from build123d import *

# Parameters (mm, degrees)
SKETCH1_R           = 3
BOSS_EXTRUDE1_DEPTH = 2
FILLET1_R           = 2


with BuildPart() as part:
    # Sketch1 → Boss-Extrude1 (new, symmetric)
    with BuildSketch(Plane(origin=(0, 0, 0), x_dir=(1, 0, 0), z_dir=(0, 1, 0))):
        with BuildLine():
            Line((0, -7.5), (180, -7.5))
            ThreePointArc((180, -7.5), (183, -4.5), (180, -1.5))
            Line((180, -1.5), (7.348469228, -1.5))
            ThreePointArc((7.348469228, -1.5), (-4.74341649, 5.809475019), (0, -7.5))
        make_face()
        with Locations(Location((0, 0, 0), (0, 0, 270))):
            Circle(SKETCH1_R, mode=Mode.SUBTRACT)
    extrude(amount=BOSS_EXTRUDE1_DEPTH, both=True)

    # Fillet1
    fillet1_edges = [part.edges().sort_by_distance(p)[0] for p in [
        (7.348469228, 0, 1.5),
    ]]
    fillet(fillet1_edges, radius=FILLET1_R)


solid = part.part
Geometry: final body of the model. Coordinates: model frame, mm. A direction names the side the tool comes from. Round coordinates to 2 decimals unless told otherwise and drop trailing zeros. Write each loop counter-clockwise with the first axis right and the second up, starting at its lowest first coordinate (ties: lowest second). Pieces come first, ordered by that corner, then holes. Notation, with made-up numbers: M 59,-11.75 L 118,-11.75 A20 cw 118,7.25 Z; hole C -8,85 d7. An arc over 180 degrees is marked long. Write item = value, one per line.
Item 1: Material intervals for line 1 along Z through (x, y) = (79.5, -0.1); line 2 along X through (y, z) = (0.4, 0); line 3 along X through (y, z) = (1.55, -0.75), sorted ascending. Write a range as [from, to].
Findings:
line_1 = [1.5, 7.5]
line_2 = [-7.5, -3], [3, 7.55]
line_3 = [-7.46, -2.9], [2.9, 7.46]
Item 2: Pull-direction query (X, two-part tool) for faces 3 (the face through (-5.27, 0.028, -5.337)), 4 (the face through (0.9, -0.03, 2.86)), 5 (the face through (183, 0, 4.6)), 6 (the face through (86, 2, 3)); classes: pulls with the +X half, pulls with the -X half, needs draft (parallel to the pull), parting line crosses it, or undercut.
Findings:
face_3 = parting line crosses it
face_4 = undercut
face_5 = pulls with the +X half
face_6 = needs draft
Item 3: Access query for faces 1 (the face through (96, 0, 1.5)), 2 (the face through (89, 0, 7.5)). Directions: +Z, -Z, +X, -X, +Y, -Y. A direction counts if a zero-diameter tool reaches every point of the face in a straight line with its end or side. Return the directions, or none.
Findings:
face_1 = -Z, +X, +Y, -Y
face_2 = +Z, +X, -X, +Y, -Y
Item 4: Pin query (flat end, axial travel): P1, Ø1, axis at x = 126.5, y = 0, coming from the -Z side; P2, Ø1, axis at y = 1, z = -4.5, coming from the -X side; P3, Ø1, axis at y = 0.5, z = -1, coming from the +X side. Return the tip coordinate at first contact, or that it passes through.
Findings:
P1 = 1.5
P2 = -6.34
P3 = 7.48
Item 5: Section query B-B on x = 94. Return loops of the section in (y, z).
Findings:
outline = M -2,1.5 L 2,1.5 L 2,7.5 L -2,7.5 Z
Item 6: Section query A-A on y = -0.25. Return loops of the section in (x, z).
Findings:
outline = M 0,7.5 A7.5 ccw long 7.49,-0.39 A2 cw 9.49,1.5 L 180,1.5 A3 ccw 180,7.5 Z; hole C 0,0 d6
